CAD build for the part. Positions are in the model's coordinates, mm. A direction names the side the tool comes from. Give positions to 0.01 mm unless a question says otherwise; leave off trailing zeros. Write each loop counter-clockwise with the first axis right and the second up, starting at its lowest first coordinate (ties: lowest second). Pieces come first, ordered by that corner, then holes. Notation, with made-up numbers: M 38.5,89 L 89.5,89 A23 ccw 89.5,109 Z; hole C 22,-11 d11. An arc over 180 degrees is marked long. One line per question, with ' | ' between items. Start each with the question number.
1. Which spindle directions (+Z, -Z, +X, -X, +Y, -Y) get a long thin tool onto all of the face, cutting with end or side? Do faces 4 (the face through (44, 6, 4.066)), 5 (the face through (-18.653, 2.465, -31.724)), 6 (the face through (-90, 2, -17)), 7 (the face through (-87.221, 1.587, -6.822)), 8 (the face through (-83, 6, 5.066)). Say none if no direction does.
2. Cut at A-A, the plane y = 2.5. Count the separate pieces of the cut face and the enclosed holes in it, then the cut area to 3 significant figures.
3. Cut at C-C, the plane x = -39. Write the cut outline in (y, z).
4. Pull direction Y, two halves, no side cores. Call faces 1 (the face through (-20, 0, 1)), 2 (the face through (-79.493, 2, 15)), 3 (the face through (50.86, 3.7, 31.09)): released by +Y, released by -Y, zero draft, split by the parting line, or undercut.
5. Flat gauge pins, fed straight in: pin 1 (1.5 mm diameter, centred on y = 3, z = -6, fed in from +X); pin 2 (6 mm diameter, centred on x = -23.5, z = -23.5, fed in from -Y); pin 3 (1.5 mm diameter, centred on y = 5.5, z = 24.5, fed in from -X); pin 4 (1 mm diameter, centred on x = -59, y = -1.5, fed in from -Z). Where does each tip first touch, or does it go through?
6. Wall check: L1, parallel to Y at x = -66.5, z = -34; L2, parallel to X at y = 1.75, z = 17; L3, parallel to X at y = -1, z = 26. Give the ranges that are in metal, low to high.
7. Cut at B-B, the plane z = 7. Write the cut outline in (x, y).
8. Cut at D-D, the plane z = -25.5. Write the cut outline in (x, y), then the cut area to 3 significant figures.
```python
from build123d import *

# Parameters (mm, degrees)
EXTRUDE_1_DEPTH          = 5
SKETCH_3_R               = 7
SKETCH_3_R_2             = 1.5
EXTRUDE_2_DEPTH          = 80
CUT_EXTRUDE_1_DEPTH      = 80
CUT_EXTRUDE_1_DEPTH_BACK = 80
SKETCH_4_W               = 13.538348415
SKETCH_4_H               = 20
SKETCH_5_R               = 7
SKETCH_5_R_2             = 4
EXTRUDE_3_DEPTH          = 50
CUT_EXTRUDE_2_DEPTH      = 50
CUT_EXTRUDE_2_DEPTH_BACK = 50
SKETCH_6_W               = 13.538348415
SKETCH_6_H               = 17
SKETCH_7_R               = 4
CUT_EXTRUDE_3_DEPTH      = 32
CUT_EXTRUDE_START        = -32
SKETCH_8_R               = 4
CUT_EXTRUDE_4_DEPTH      = 32


with BuildPart() as part:
    # Sketch 1 → Extrude 1 (new body)
    with BuildSketch(Plane(origin=(0, 0, 0), x_dir=(1, 0, 0), z_dir=(0, 1, 0))):
        Polygon((-79.492600423, 46.934460888), (-79.492600423, -33.065539112), (40.507399577, -33.065539112), (40.507399577, 16.934460888), align=None)
    extrude(amount=EXTRUDE_1_DEPTH)

    # Sketch 3 → Extrude 2 (add)
    with BuildSketch(Plane.XY.offset(33.065539112)):
        with Locations((-86.030948838, 2.5)):
            Circle(SKETCH_3_R)
        with Locations((-86.030948838, 2.5)):
            Circle(SKETCH_3_R_2, mode=Mode.SUBTRACT)
    extrude(amount=-EXTRUDE_2_DEPTH)

    # Sketch 4 → Cut-Extrude 1 (cut, two sides: drawn at the far end of the back side and taken through both)
    with BuildSketch(Plane(origin=(0, 5, 0), x_dir=(1, 0, 0), z_dir=(0, 1, 0)).offset(-CUT_EXTRUDE_1_DEPTH_BACK)):
        with Locations((-86.26177463, 28.934460888)):
            Rectangle(SKETCH_4_W, SKETCH_4_H)
        with Locations((-86.26177463, -15.065539112)):
            Rectangle(SKETCH_4_W, SKETCH_4_H)
    extrude(amount=CUT_EXTRUDE_1_DEPTH + CUT_EXTRUDE_1_DEPTH_BACK, mode=Mode.SUBTRACT)

    # Sketch 5 → Extrude 3 (add)
    with BuildSketch(Plane.XY.offset(33.065539112)):
        with Locations((47.045747992, 2.5)):
            Circle(SKETCH_5_R)
        with Locations((47.045747992, 2.5)):
            Circle(SKETCH_5_R_2, mode=Mode.SUBTRACT)
    extrude(amount=-EXTRUDE_3_DEPTH)

    # Sketch 6 → Cut-Extrude 2 (cut, two sides: drawn at the far end of the back side and taken through both)
    with BuildSketch(Plane(origin=(0, 5, 0), x_dir=(1, 0, 0), z_dir=(0, 1, 0)).offset(-CUT_EXTRUDE_2_DEPTH_BACK)):
        with Locations((47.276573785, 4.434460888)):
            Rectangle(SKETCH_6_W, SKETCH_6_H)
        with Locations((47.276573785, -20.565539112)):
            Rectangle(SKETCH_6_W, SKETCH_6_H)
    extrude(amount=CUT_EXTRUDE_2_DEPTH + CUT_EXTRUDE_2_DEPTH_BACK, mode=Mode.SUBTRACT)

    # Sketch 7 → Cut-Extrude 3 (cut)
    with BuildSketch(Plane.XY.offset(33.065539112)):
        with Locations((-86.030948838, 2.5)):
            Circle(SKETCH_7_R)
    extrude(amount=-CUT_EXTRUDE_3_DEPTH, mode=Mode.SUBTRACT)

    # Sketch 8 → Cut-Extrude 4 (cut)
    with BuildSketch(Plane(origin=(0, 0, -46.934460888), x_dir=(-1, 0, 0), z_dir=(0, 0, -1)).offset(CUT_EXTRUDE_START)):
        with Locations(Location((86.030948838, 2.5, 0), (0, 0, 180))):
            Circle(SKETCH_8_R)
    extrude(amount=CUT_EXTRUDE_4_DEPTH, mode=Mode.SUBTRACT)


solid = part.part
```
Here are the results:
1) face 4: +X, +Y, -Y | face 5: -Z, +X, +Y, -Y | face 6: -Z | face 7: +Z, -Z | face 8: -X, +Y, -Y
2) separate pieces: 7 | enclosed holes: 0 | area: 8,190 mm^2
3) outline: M 0,-36.81 L 5,-36.81 L 5,33.07 L 0,33.07 Z
4) face 1: released by -Y | face 2: zero draft | face 3: undercut
5) pin 1: x = 40.51 | pin 2: y = 0 | pin 3: x = -92.57 | pin 4: through
6) L1: 0 to 5 | L2: -79.49 to 40.51 | L3: -92.09 to -87.97, -84.09 to -79.97
7) outline: M -79.49,0 L 40.51,0 A7 ccw long 40.51,5 L -79.49,5 Z; hole C 47.05,2.5 d8
8) outline: M -79.49,0 L 6.25,0 L 6.25,5 L -79.49,5 Z | area: 429 mm^2
